from build123d import *

# Parameters (mm, degrees)
F0_W     = 65
F0_H     = 30
F1_DEPTH = 1.35
F2_W     = 12.75
F2_H     = 11.9
F2_W_2   = 2.55
F3_DEPTH = 1.5
F2_W_3   = 7.8
F2_H_2   = 4.5
F2_H_3   = 1
F4_DEPTH = 1.5
F2_W_4   = 1
F2_H_4   = 16.8
F2_W_5   = 3.4
F5_DEPTH = 1
F2_W_6   = 11.2
F2_H_5   = 0.5
F2_H_6   = 7
F6_DEPTH = 3.2
F7_D     = 3.3
F7_DEPTH = 9
F7_TIP   = 0.9914200214


with BuildPart() as f1:
    # F0 (on Top) → F1 (new body)
    with BuildSketch(Plane.XY):
        Rectangle(F0_W, F0_H)
    extrude(amount=F1_DEPTH)

    # F2 (on face) → F3 (join)
    with BuildSketch(Plane.XY.offset(1.35)):
        with Locations((26.125, -1.55)):
            Rectangle(F2_W, F2_H)
        with Locations((33.775, -1.55)):
            Rectangle(F2_W_2, F2_H)
    extrude(amount=F3_DEPTH)

    # F2 (on face) → F4 (join)
    with BuildSketch(Plane.XY.offset(1.35)):
        with Locations((-21.6, 12.75)):
            Rectangle(F2_W_3, F2_H_2)
        with Locations((-8.6, 15.5)):
            Rectangle(F2_W_3, F2_H_3)
        with Locations((-8.6, 12.75)):
            Rectangle(F2_W_3, F2_H_2)
        with Locations((-21.6, 15.5)):
            Rectangle(F2_W_3, F2_H_3)
    extrude(amount=F4_DEPTH)

    # F2 (on face) → F5 (join)
    with BuildSketch(Plane.XY.offset(1.35)):
        with Locations((-33, -0.1)):
            Rectangle(F2_W_4, F2_H_4)
        with Locations((-30.8, -0.1)):
            Rectangle(F2_W_5, F2_H_4)
    extrude(amount=F5_DEPTH)

    # F2 (on face) → F6 (join)
    with BuildSketch(Plane.XY.offset(1.35)):
        with Locations((19.7, 15.25)):
            Rectangle(F2_W_6, F2_H_5)
        with Locations((19.7, 11.5)):
            Rectangle(F2_W_6, F2_H_6)
    extrude(amount=F6_DEPTH)

    # F7
    with Locations(Plane.XY.offset(1.35)):
        with Locations((28.5, 11), (28.5, -11), (-28.5, 11), (-28.5, -11)):
            Hole(F7_D / 2, depth=F7_DEPTH)
            with Locations((0, 0, -(F7_DEPTH + F7_TIP / 2))):  # 118° drill point
                Cone(0, F7_D / 2, F7_TIP, mode=Mode.SUBTRACT)


solid = f1.part
Work out the finished part from the listing and answer in its coordinate system (mm). A direction names the side the tool comes from. Give positions to 0.01 mm unless a question says otherwise; leave off trailing zeros. Order: outer loops, then holes, each group sorted by start corner. A loop starts at its lowest first (then second) coordinate and runs counter-clockwise, first axis right, second up. Notation, with made-up numbers: (-18, 46.25) -> (7, 46.25) arc R24 ccw to (7, 57.25) -> close; hole circle Ø11 at (61, 10.5). An arc over 180 degrees is marked (long way). Answer as a JSON object with one key per item and string values. Group by question number.
1. Section C-C on y = 0 is taken. Determine the outline of the cut face in (x, z), plus the area to 3 significant figures.
2. Section A-A on x = 28.5 is taken. Determine the outline of the cut face in (y, z).
3. Consider line 1 along Y through (x, z) = (28.5, 0.75); line 2 along Y through (x, z) = (20, 2.45); line 3 along Z through (x, y) = (-1, 5). Determine where each line is inside the solid, lowest interval first. Write a range as [from, to].
4. Section B-B on y = -11 is taken. Determine the outline of the cut face in (x, z).
5. Section D-D on x = -21 is taken. Determine the outline of the cut face in (y, z).
6. A tool of negligible diameter and unlimited length cuts with its end or side. For faces 5 (the flat face through (19.75, -2, 2)), 6 (the flat face through (25.3, 12, 3)), 7 (the flat face through (27, -7.5, 2)), 8 (the flat face through (-31, 0, 2.35)), 9 (the flat face through (-4.7, 13, 2)), from which of +Z, -Z, +X, -X, +Y, -Y can it reach the whole face along a straight path? Write none if from no direction.
7. Flat-ended cylindrical pins translate along their axes: pin 1 Ø1 at (x, y) = (-9, 12) entering from +Z; pin 2 Ø1 at (x, z) = (6.5, 3.5) entering from -Y; pin 3 Ø1.6 at (x, z) = (-22, 2.5) entering from -Y; pin 4 Ø1.3 at (x, y) = (34, 0.5) entering from -Z. Find the tip coordinate at first contact, or state that the pin passes through.
8. The mould has two halves that part along X. Classify faces 1 (the cylindrical face through (29.81, -12, 0.67)), 2 (the flat face through (35.05, -2, 2)), 3 (the cylindrical face through (29.81, 10, 0.67)), 4 (the flat face through (34, -1, 1.35)): released by +X, released by -X, zero draft, split by the parting line, or undercut.
Result sheet:
{
 "1": {"outline": "(-33.5, 1.35) -> (-32.5, 1.35) -> (-32.5, 0) -> (32.5, 0) -> (32.5, 1.35) -> (35.05, 1.35) -> (35.05, 2.85) -> (19.75, 2.85) -> (19.75, 1.35) -> (-29.1, 1.35) -> (-29.1, 2.35) -> (-33.5, 2.35) -> close", "area": "115 mm^2"},
 "2": {"outline": "(-15, 0) -> (-12.65, 0) -> (-12.65, 1.35) -> (-15, 1.35) -> close; (-9.35, 0) -> (9.35, 0) -> (9.35, 1.35) -> (4.4, 1.35) -> (4.4, 2.85) -> (-7.5, 2.85) -> (-7.5, 1.35) -> (-9.35, 1.35) -> close; (12.65, 0) -> (15, 0) -> (15, 1.35) -> (12.65, 1.35) -> close"},
 "3": {"line 1": "y = [-15, -12.65], [-9.35, 9.35], [12.65, 15]", "line 2": "y = [-7.5, 4.4], [8, 15.5]", "line 3": "z = [0, 1.35]"},
 "4": {"outline": "(-32.5, 0) -> (-30.15, 0) -> (-30.15, 1.35) -> (-32.5, 1.35) -> close; (-26.85, 0) -> (26.85, 0) -> (26.85, 1.35) -> (-26.85, 1.35) -> close; (30.15, 0) -> (32.5, 0) -> (32.5, 1.35) -> (30.15, 1.35) -> close"},
 "5": {"outline": "(-15, 0) -> (15, 0) -> (15, 1.35) -> (16, 1.35) -> (16, 2.85) -> (10.5, 2.85) -> (10.5, 1.35) -> (-15, 1.35) -> close"},
 "6": {"face 5": "+Z, -Y", "face 6": "+Z, +X, +Y", "face 7": "+Z, +X, -Y", "face 8": "+Z, -X, +Y, -Y", "face 9": "+Z, +Y, -Y"},
 "7": {"pin 1": "stops at z = 2.85", "pin 2": "passes through", "pin 3": "stops at y = 10.5", "pin 4": "stops at z = 1.35"},
 "8": {"face 1": "undercut", "face 2": "released by +X", "face 3": "undercut", "face 4": "zero draft"}
}
